from build123d import *

# Parameters (mm, degrees)
F0_W        = 90
F0_H        = 60
F1_DEPTH    = 2.5
F2_W        = 95
F2_H        = 65
F2_W_2      = 90
F2_H_2      = 60
F3_DEPTH    = 10
F4_T1_DEPTH = 7.5
F5_T1_DEPTH = 65
F6_R        = 3
F7_DEPTH    = 10
F10_R       = 6.1
F11_DEPTH   = 6
F12_R       = 10


# Not quite as in the source:
# - a fillet or chamfer that OpenCascade refuses, or shapes differently, is made with other operations: its cross-section is extruded or revolved along the edge and cut away or added


with BuildPart() as f1:
    # F0 (on Top) → F1 (new body)
    with BuildSketch(Plane.XY):
        Rectangle(F0_W, F0_H)
    extrude(amount=F1_DEPTH)

    # F2 (on Top) → F3 (join)
    with BuildSketch(Plane.XY):
        Rectangle(F2_W, F2_H)
        Rectangle(F2_W_2, F2_H_2, mode=Mode.SUBTRACT)
    extrude(amount=F3_DEPTH)

    # F4: fillet of radius 10 on 4 edges, made by hand

    # F4_s2 → F4_t1 (join)
    with BuildSketch(Plane.XY.offset(2.5)):
        with BuildLine():
            add(Edge.make_bspline(
                [(-45, 20), (-45, 30), (-35, 30)],
                knots=[0, 0, 0, 1, 1, 1], degree=2, weights=[1, 1.5, 1]))
            Line((-35, 30), (-45, 30))
            Line((-45, 30), (-45, 20))
        make_face()
        with BuildLine():
            add(Edge.make_bspline(
                [(45, 20), (45, 30), (35, 30)],
                knots=[0, 0, 0, 1, 1, 1], degree=2, weights=[1, 1.5, 1]))
            Line((35, 30), (45, 30))
            Line((45, 30), (45, 20))
        make_face()
        with BuildLine():
            add(Edge.make_bspline(
                [(45, -20), (45, -30), (35, -30)],
                knots=[0, 0, 0, 1, 1, 1], degree=2, weights=[1, 1.5, 1]))
            Line((35, -30), (45, -30))
            Line((45, -30), (45, -20))
        make_face()
        with BuildLine():
            add(Edge.make_bspline(
                [(-35, -30), (-45, -30), (-45, -20)],
                knots=[0, 0, 0, 1, 1, 1], degree=2, weights=[1, 1.5, 1]))
            Line((-45, -20), (-45, -30))
            Line((-45, -30), (-35, -30))
        make_face()
    extrude(amount=F4_T1_DEPTH)

    # F5: fillet of radius 11 on 4 edges, made by hand

    # F5_s2 → F5_t1 (cut)
    with BuildSketch(Plane.XY.offset(-27.5)):
        with BuildLine():
            add(Edge.make_bspline(
                [(-36.5, 32.5), (-47.5, 32.5), (-47.5, 21.5)],
                knots=[0, 0, 0, 1, 1, 1], degree=2, weights=[1, 1.5, 1]))
            Line((-47.5, 21.5), (-47.5, 32.5))
            Line((-47.5, 32.5), (-36.5, 32.5))
        make_face()
        with BuildLine():
            add(Edge.make_bspline(
                [(-36.5, -32.5), (-47.5, -32.5), (-47.5, -21.5)],
                knots=[0, 0, 0, 1, 1, 1], degree=2, weights=[1, 1.5, 1]))
            Line((-47.5, -21.5), (-47.5, -32.5))
            Line((-47.5, -32.5), (-36.5, -32.5))
        make_face()
        with BuildLine():
            add(Edge.make_bspline(
                [(47.5, 21.5), (47.5, 32.5), (36.5, 32.5)],
                knots=[0, 0, 0, 1, 1, 1], degree=2, weights=[1, 1.5, 1]))
            Line((36.5, 32.5), (47.5, 32.5))
            Line((47.5, 32.5), (47.5, 21.5))
        make_face()
        with BuildLine():
            add(Edge.make_bspline(
                [(36.5, -32.5), (47.5, -32.5), (47.5, -21.5)],
                knots=[0, 0, 0, 1, 1, 1], degree=2, weights=[1, 1.5, 1]))
            Line((47.5, -21.5), (47.5, -32.5))
            Line((47.5, -32.5), (36.5, -32.5))
        make_face()
    extrude(amount=F5_T1_DEPTH, mode=Mode.SUBTRACT)

    # F6 (on face) → F7 (join)
    with BuildSketch(Plane.XY.offset(2.5)):
        with Locations((-40, 24.5)):
            Circle(F6_R)
        with Locations((-40, -24.5)):
            Circle(F6_R)
        with Locations((18, -24.5)):
            Circle(F6_R)
        with Locations((18, 24.5)):
            Circle(F6_R)
    extrude(amount=F7_DEPTH)

    # F10 (on offset) → F11 (join)
    with BuildSketch(Plane(origin=(0, 11, 0), x_dir=(-1, 0, 0), z_dir=(0, 1, 0))):
        with BuildLine():
            Line((45, 0), (47.5, 0))
            Line((47.5, 0), (54.148522424, 8.0868878322))
            Line((54.148522424, 8.0868878322), (54.148522424, 33.5947699827))
            Line((54.148522424, 33.5947699827), (50.6855217688, 38.5))
            ThreePointArc((50.6855217688, 38.5), (41.5427608844, 47.6427608844), (32.4, 38.5))
            Line((32.4, 38.5), (32.4, 34.8039232194))
            Line((32.4, 34.8039232194), (42.2389033973, 22.7499233782))
            Line((42.2389033973, 22.7499233782), (45, 12.8317605704))
            Line((45, 12.8317605704), (45, 0))
        make_face()
        with Locations((41.5, 38.5)):
            Circle(F10_R, mode=Mode.SUBTRACT)
    extrude(amount=F11_DEPTH)

    # F12
    f12_edges = [f1.edges().sort_by_distance(p)[0] for p in [
        (-32.4, 14, 34.803923),
        (-42.238903, 14, 22.749923),
        (-45, 14, 12.831761),
        (-50.685522, 14, 38.5),
        (-54.148522, 14, 33.59477),
        (-54.148522, 14, 8.086888),
    ]]
    fillet(f12_edges, radius=F12_R)


solid = f1.part
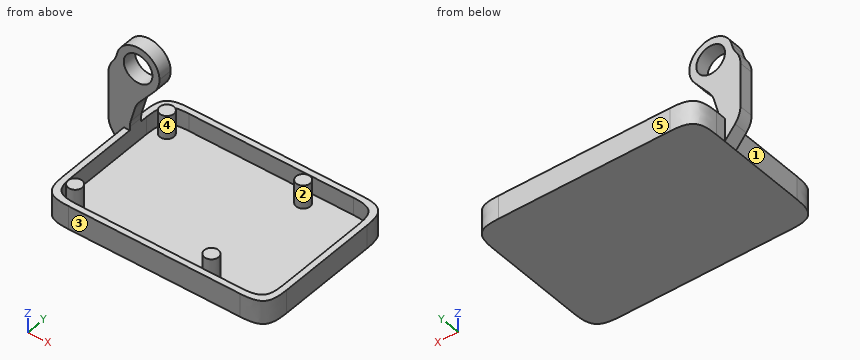
Geometry check sheet. Reference: the model listing, model coordinates, mm. Face numbers are marked on the shaded views. A direction names the side the tool comes from. Coordinates: 2 decimals unless noted, no trailing zeros. Order: outer loops, then holes, each group sorted by start corner. A loop starts at its lowest first (then second) coordinate and runs counter-clockwise, first axis right, second up. Notation, with made-up numbers: (46.5, 29.5) -> (85.5, 29.5) arc R30 ccw to (85.5, 52.5) -> close; hole circle Ø7 at (28.5, 81). An arc over 180 degrees is marked (long way). Use a Markdown table: item, result. Add a question column.
1. Material ranges on L1, parallel to Y at x = -25.5, z = 6; L2, parallel to Z at x = -41.5, y = 13.15; L3, parallel to Z at x = -41, y = 14, recorded low to high.
2. Set-up check for the marked faces 4 and 5: record each of +Z, -Z, +X, -X, +Y, -Y from which the full face is reachable in a straight line by a thin tool's end or side.
3. Go/stop test with flat-tipped pins: pin 1 Ø19.5 at (x, y) = (22, -3) entering from +Z; pin 2 Ø8 at (y, z) = (-10.5, 6) entering from -X; pin 3 Ø24 at (x, z) = (-45.5, 33) entering from +Y; pin 4 Ø3 at (x, y) = (5.5, -22) entering from -Z. Record where each tip stops, or that it passes through.
4. Cross-section at A-A (y = -18.5). Enter the section's corners in (x, z).
5. Cross-section at C-C (z = 8). Give the number of separate pieces and of enclosed holes in the cut face, and give its area (3 significant figures).
6. Cross-section at D-D (z = 29). Enter the section's corners in (x, y), and give its area (3 significant figures).
7. Cross-section at B-B (x = -14). Enter the section's corners in (y, z), and give its area (3 significant figures).
8. Mould release check, pull along Y, two halves, no side actions. Record for the marked faces 1, 2 and 3: pulls with the +Y half, pulls with the -Y half, needs draft (parallel to the pull), parting line crosses it, or undercut.
Filled sheet:
| question | item | result |
|---|---|---|
| 1 | L1 | -32.5 to -30, 30 to 32.5 |
| 1 | L2 | 0 to 2.5, 23.58 to 32.4, 44.6 to 47.64 |
| 1 | L3 | 0 to 2.5, 24.27 to 32.42, 44.58 to 47.63 |
| 2 | face 4 | +Z |
| 2 | face 5 | +Z, -Z, +X, -X, +Y |
| 3 | pin 1 | z = 2.5 |
| 3 | pin 2 | x = -47.5 |
| 3 | pin 3 | y = 17 |
| 3 | pin 4 | z = 0 |
| 4 | outline | (-47.5, 0) -> (47.5, 0) -> (47.5, 10) -> (45, 10) -> (45, 2.5) -> (-45, 2.5) -> (-45, 10) -> (-47.5, 10) -> close |
| 5 | separate pieces | 5 |
| 5 | enclosed holes | 1 |
| 5 | area | 914 mm2 |
| 6 | outline | (-54.15, 11) -> (-37.14, 11) -> (-37.14, 17) -> (-54.15, 17) -> close |
| 6 | area | 102 mm2 |
| 7 | outline | (-32.5, 0) -> (32.5, 0) -> (32.5, 10) -> (30, 10) -> (30, 2.5) -> (-30, 2.5) -> (-30, 10) -> (-32.5, 10) -> close |
| 7 | area | 200 mm2 |
| 8 | face 1 | needs draft |
| 8 | face 2 | undercut |
| 8 | face 3 | pulls with the -Y half |
